The model under review builds one solid part; all positions refer to its coordinate system, in mm. A direction names the side the tool comes from. Round coordinates to 2 decimals unless told otherwise and drop trailing zeros. Order: outer loops, then holes, each group sorted by start corner. A loop starts at its lowest first (then second) coordinate and runs counter-clockwise, first axis right, second up.
```python
from build123d import *

# Parameters (mm, degrees)
SKETCH1_R               = 15
SKETCH1_R_2             = 3.5
BOSS_EXTRUDE2_DEPTH     = 5
CUT_EXTRUDE5_DEPTH      = 83.400646631
CUT_EXTRUDE5_DEPTH_BACK = 83.400646631
CUT_EXTRUDE6_DEPTH      = 83.400646631
CUT_EXTRUDE6_DEPTH_BACK = 83.400646631


with BuildPart() as part:
    # Sketch1 → Boss-Extrude2 (new body)
    with BuildSketch(Plane.XY):
        with BuildLine():
            ThreePointArc((-25.586643761, 21.659966753), (-25.54707355, 21.487234362), (-25.502809349, 21.315644849))
            Line((-25.502809349, 21.315644849), (-18.331305953, -4.996320852))
            ThreePointArc((-18.331305953, -4.996320852), (-1.350797033, -18.951921997), (17.437371999, -7.545731095))
            Line((17.437371999, -7.545731095), (44.790602171, 55.664638301))
            ThreePointArc((44.790602171, 55.664638301), (44.35983755, 61.654536494), (39.204715036, 64.734982954))
            Line((39.204715036, 64.734982954), (-27.25170969, 68.621949973))
            ThreePointArc((-27.25170969, 68.621949973), (-32.565561595, 66.364169918), (-33.986309951, 60.768093886))
            Line((-33.986309951, 60.768093886), (-25.586643761, 21.659966753))
        make_face()
        Circle(SKETCH1_R, mode=Mode.SUBTRACT)
        with Locations((-19.231573102, 23.024912509)):
            Circle(SKETCH1_R_2, mode=Mode.SUBTRACT)
        with Locations((-27.631239292, 62.133039642)):
            Circle(SKETCH1_R_2, mode=Mode.SUBTRACT)
        with Locations((38.825185434, 58.246072623)):
            Circle(SKETCH1_R_2, mode=Mode.SUBTRACT)
    extrude(amount=BOSS_EXTRUDE2_DEPTH)

    # Sketch7 → Cut-Extrude5 (cut, two sides: drawn at the far end of the back side and taken through both)
    with BuildSketch(Plane.XY.offset(-CUT_EXTRUDE5_DEPTH_BACK)):
        with BuildLine():
            Line((-24.243201443, 51.12071929), (-20.237707665, 32.471482957))
            ThreePointArc((-20.237707665, 32.471482957), (-16.449923424, 32.108547523), (-13.108406148, 30.288301969))
            ThreePointArc((-13.108406148, 30.288301969), (-8.731595333, 32.674535637), (-4.738186305, 35.658370146))
            ThreePointArc((-4.738186305, 35.658370146), (-3.700454424, 37.933841025), (-4.747603131, 40.204993764))
            Line((-4.747603131, 40.204993764), (-20.251388243, 53.499512061))
            ThreePointArc((-20.251388243, 53.499512061), (-21.600184602, 54.086137653), (-23.045406965, 53.812799907))
            ThreePointArc((-23.045406965, 53.812799907), (-24.083058347, 52.661975629), (-24.243201443, 51.12071929))
        make_face()
    extrude(amount=CUT_EXTRUDE5_DEPTH + CUT_EXTRUDE5_DEPTH_BACK, mode=Mode.SUBTRACT)

    # Sketch7_3 → Cut-Extrude6 (cut, two sides: drawn at the far end of the back side and taken through both)
    with BuildSketch(Plane.XY.offset(-CUT_EXTRUDE6_DEPTH_BACK)):
        with BuildLine():
            Line((-17.973069241, 56.156439333), (-2.469284129, 42.861921035))
            ThreePointArc((-2.469284129, 42.861921035), (-0.064983066, 42.173450574), (2.025573232, 43.546122983))
            ThreePointArc((2.025573232, 43.546122983), (4.977414301, 49.417863243), (6.779548794, 55.737911554))
            ThreePointArc((6.779548794, 55.737911554), (6.192076358, 58.135617799), (4.005220181, 59.280947081))
            Line((4.005220181, 59.280947081), (-16.230971238, 60.464540827))
            ThreePointArc((-16.230971238, 60.464540827), (-17.729787246, 60.071141831), (-18.708849124, 58.870038157))
            ThreePointArc((-18.708849124, 58.870038157), (-18.758574348, 57.400004307), (-17.973069241, 56.156439333))
        make_face()
        with BuildLine():
            Line((16.843883891, 46.763721743), (28.352089566, 53.85127309))
            ThreePointArc((28.352089566, 53.85127309), (29.281554059, 54.870744477), (29.52876331, 56.227989384))
            ThreePointArc((29.52876331, 56.227989384), (28.676191314, 57.411652758), (27.308139041, 57.917983644))
            Line((27.308139041, 57.917983644), (13.941676384, 58.699774114))
            ThreePointArc((13.941676384, 58.699774114), (12.198740022, 58.263103257), (11.01733755, 56.909294999))
            ThreePointArc((11.01733755, 56.909294999), (10.906611403, 56.14688363), (10.780846845, 55.386808205))
            ThreePointArc((10.780846845, 55.386808205), (11.390405083, 51.765860667), (12.465443048, 48.254861422))
            ThreePointArc((12.465443048, 48.254861422), (14.303549595, 46.47831417), (16.843883891, 46.763721743))
        make_face()
        with BuildLine():
            ThreePointArc((18.040522196, 39.202488559), (20.980340559, 36.423565175), (24.287649202, 34.094046616))
            ThreePointArc((24.287649202, 34.094046616), (26.280456073, 33.862297186), (27.766942681, 35.209644428))
            Line((27.766942681, 35.209644428), (33.348917717, 48.108987643))
            ThreePointArc((33.348917717, 48.108987643), (33.512477865, 49.558438608), (32.839288491, 50.852454099))
            ThreePointArc((32.839288491, 50.852454099), (31.516061413, 51.242367015), (30.18747827, 50.871113983))
            Line((30.18747827, 50.871113983), (18.679272595, 43.783562635))
            ThreePointArc((18.679272595, 43.783562635), (17.281206586, 41.643430104), (18.040522196, 39.202488559))
        make_face()
        with BuildLine():
            ThreePointArc((5.483845255, 41.532282971), (3.820360163, 39.072317803), (1.974521731, 36.746056477))
            ThreePointArc((1.974521731, 36.746056477), (-1.572739771, 33.116585642), (-5.561267488, 29.978470067))
            ThreePointArc((-5.561267488, 29.978470067), (-7.422805487, 24.125679952), (-2.206440861, 20.883764477))
            ThreePointArc((-2.206440861, 20.883764477), (6.856161822, 19.849258048), (14.625251307, 15.069904585))
            ThreePointArc((14.625251307, 15.069904585), (17.298768965, 14.280178644), (19.467842186, 16.031316872))
            Line((19.467842186, 16.031316872), (23.370103648, 25.049022897))
            ThreePointArc((23.370103648, 25.049022897), (23.564224135, 28.492082606), (21.483147911, 31.241894358))
            ThreePointArc((21.483147911, 31.241894358), (15.918845504, 35.767827579), (11.498679992, 41.416515006))
            Line((11.498679992, 41.416515006), (11.497097402, 41.415540337))
            ThreePointArc((11.497097402, 41.415540337), (11.469933131, 41.462392803), (11.442047157, 41.508819343))
            ThreePointArc((11.442047157, 41.508819343), (8.469494844, 43.183469976), (5.483845255, 41.532282971))
        make_face()
    extrude(amount=CUT_EXTRUDE6_DEPTH + CUT_EXTRUDE6_DEPTH_BACK, mode=Mode.SUBTRACT)


solid = part.part
```
(1) Consider section C-C (z = 2.85). State how many separate pieces and enclosed holes the cut face has, and give its area (3 significant figures).
Data:
separate pieces: 1
enclosed holes: 9
area: 2,510 mm2
(2) Consider section B-B (y = 8.5). Write out the cut boundary in (x, z), and give its area (3 significant figures).
Data:
outline: (-22.01, 0) - (-12.36, 0) - (-12.36, 5) - (-22.01, 5) - close; (12.36, 0) - (24.38, 0) - (24.38, 5) - (12.36, 5) - close
area: 108 mm2
(3) Draft analysis for pull direction Y (two halves, no side actions). For faces 3 (the flat face through (21.4, 20.5, 2.5)), 4 (the flat face through (30.923, 23.617, 2.465)), state which applies: pulls with the +Y half, pulls with the -Y half, needs draft (parallel to the pull), parting line crosses it, or undercut.
Data:
face 3: undercut
face 4: pulls with the -Y half
(4) Insertion check: pin 1 (3 mm diameter, centred on x = -4, z = 1, fed in from -Y); pin 2 (1.5 mm diameter, centred on x = -22, z = 1.5, fed in from +Y); pin 3 (3 mm diameter, centred on x = 37, z = 2.5, fed in from +Y). Each pin has a flat end and moves straight along its axis. Give the tip position at first contact, or say it passes through.
Data:
pin 1: stops at y = -18.83
pin 2: stops at y = 68.36
pin 3: stops at y = 64.95
(5) For faces 1 (the cylindrical face through (-1.678, -18.926, 2.465)), 2 (the flat face through (24.514, 47.377, 2.465)), list the 3-axis set-ups (+Z, -Z, +X, -X, +Y, -Y) from which the entire face can be reached by the end or side of a thin tool; tool diameter is ignored.
Data:
face 1: +Z, -Z, -Y
face 2: +Z, -Z
(6) To check wall thickness, follow probe 1 along X at (y, z) = (23.5, 3.6); probe 2 along Y at (x, z) = (-11.5, 2.2); probe 3 along Y at (x, z) = (-11, 2). State the ranges of each line that lie inside material, in increasing order.
Data:
probe 1: x = -25.98 to -22.7, -15.76 to -7.14, 22.7 to 30.87
probe 2: y = -15.12 to -9.63, 9.63 to 31.07, 46 to 50.61, 60.19 to 67.7
probe 3: y = -15.49 to -10.2, 10.2 to 31.34, 45.57 to 50.18, 60.16 to 67.67
(7) Consider section A-A (x = 0). Write out the cut boundary in (y, z).
Data:
outline: (-19, 0) - (-15, 0) - (-15, 5) - (-19, 5) - close; (15, 0) - (21, 0) - (21, 5) - (15, 5) - close; (34.61, 0) - (42.18, 0) - (42.18, 5) - (34.61, 5) - close; (59.52, 0) - (67.03, 0) - (67.03, 5) - (59.52, 5) - close
